Geometry: final body of the model. Coordinates: model frame, mm. Coordinates: 2 decimals unless noted, no trailing zeros. Write each loop counter-clockwise with the first axis right and the second up, starting at its lowest first coordinate (ties: lowest second). Pieces come first, ordered by that corner, then holes. Notation, with made-up numbers: (44.25, 52) - (60.25, 52) arc R21 ccw to (60.25, 87) - close; hole circle Ø5 at (75, 42.25). An arc over 180 degrees is marked (long way). Put each result on its own line as item: value.
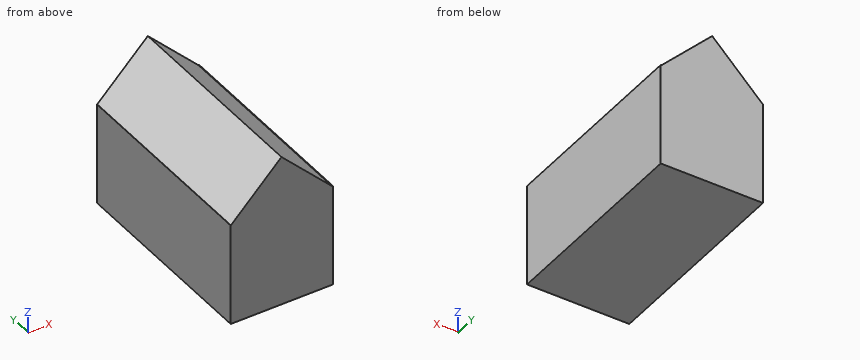
```python
from build123d import *

# Parameters (mm, degrees)
BOX001_W               = 7
BOX001_H               = 20
BOX001_DEPTH           = 7.05
BOX001_PLACEMENT_ANGLE = 45
BOX_W                  = 10
BOX_H                  = 20
BOX_DEPTH              = 10


with BuildPart() as cub001:
    # Box001 → Box001 (new body)
    with BuildSketch(Plane.XY):
        with Locations((3.5, 10)):
            Rectangle(BOX001_W, BOX001_H)
    extrude(amount=BOX001_DEPTH)


with BuildPart() as cub001_1:
    # Box001 placement: moved
    add(cub001.part.moved(Location((5, 0, 5.03))).rotate(Axis((5, 0, 5.03), (0, -1, 0)), BOX001_PLACEMENT_ANGLE))


with BuildPart() as fusion:
    # Box → Box (new body)
    with BuildSketch(Plane.XY):
        with Locations((5, 10)):
            Rectangle(BOX_W, BOX_H)
    extrude(amount=BOX_DEPTH)

    # Fusion: union Cub001
    add(cub001_1.part)


solid = fusion.part
```
1. Ray query, probe 1 along X at (y, z) = (9.5, 14); probe 2 along X at (y, z) = (15.25, 13.25); probe 3 along Z at (x, y) = (1.5, 2.5). Return the intervals inside material, ascending. Write a range as from..to.
Answer below:
probe 1: x = 4..5.93
probe 2: x = 3.25..6.68
probe 3: z = 0..11.5
2. Section query B-B (x = 6). Return loops of the section in (y, z), then the cut area to 3 significant figures.
Answer below:
outline: (0, 0) - (20, 0) - (20, 13.93) - (0, 13.93) - close
area: 279 mm²
3. Section query C-C (z = 12.25). Return loops of the section in (x, y), then the cut area to 3 significant figures.
Answer below:
outline: (2.25, 0) - (7.68, 0) - (7.68, 20) - (2.25, 20) - close
area: 109 mm²
4. Pin query (flat end, axial travel): pin 1 Ø5 at (x, y) = (6, 4.5) entering from +Z. Return the tip coordinate at first contact, or that it passes through.
Answer below:
pin 1: stops at z = 14.96
